Can you work these out from the model? Positions are in its coordinate system, mm. A direction names the side the tool comes from. Coordinates: 2 decimals unless noted, no trailing zeros. Write each loop counter-clockwise with the first axis right and the second up, starting at its lowest first coordinate (ties: lowest second). Pieces come first, ordered by that corner, then holes. Notation, with made-up numbers: M -21,67.5 L -1,67.5 A8 ccw -1,80.5 Z; hole C -5,1.5 d9. An arc over 180 degrees is marked long. Use one line per item in the form item = value. Start each with the question number.
```python
from build123d import *

# Parameters (mm, degrees)
SKETCH_1_W          = 70
SKETCH_1_H          = 80
EXTRUDE_1_DEPTH     = 4
SKETCH_2_W          = 70
SKETCH_2_H          = 4
EXTRUDE_2_DEPTH     = 16
CUT_EXTRUDE_1_DEPTH = 109.166538264
CHAMFER_1_SIZE      = 20
SKETCH_8_W          = 30
SKETCH_8_H          = 3
EXTRUDE_4_DEPTH     = 34
EXTRUDE_START       = 10
EXTRUDE_6_DEPTH     = 10
SKETCH_11_W         = 9
SKETCH_11_H         = 37.243398564
CUT_EXTRUDE_2_DEPTH = 10
CHAMFER_2_SIZE      = 3
SKETCH_12_W         = 3
SKETCH_12_H         = 48
EXTRUDE_7_DEPTH     = 6
CHAMFER_3_SIZE      = 5
SKETCH_13_W         = 9
SKETCH_13_H         = 3
EXTRUDE_8_DEPTH     = 6
CHAMFER_4_SIZE      = 10
CUT_EXTRUDE_3_DEPTH = 4
FILLET_3_R          = 3
SKETCH_15_R         = 2.5
CUT_EXTRUDE_4_DEPTH = 4
FILLET_4_R          = 10
SKETCH_16_R         = 1.5
CUT_EXTRUDE_5_DEPTH = 4


with BuildPart() as part:
    # 草图1 → 凸台-拉伸1 (new body)
    with BuildSketch(Plane(origin=(0, 0, 0), x_dir=(1, 0, 0), z_dir=(0, 1, 0))):
        with Locations((35, 40)):
            Rectangle(SKETCH_1_W, SKETCH_1_H)
    extrude(amount=EXTRUDE_1_DEPTH)

    # 草图2 → 凸台-拉伸2 (add)
    with BuildSketch(Plane(origin=(0, 4, 0), x_dir=(1, 0, 0), z_dir=(0, 1, 0))):
        with Locations((35, 2)):
            Rectangle(SKETCH_2_W, SKETCH_2_H)
    extrude(amount=EXTRUDE_2_DEPTH)

    # 草图4 → 切除-拉伸1 (cut, through all)
    with BuildSketch(Plane(origin=(0, 20, 0), x_dir=(1, 0, 0), z_dir=(0, 1, 0))):
        with BuildLine():
            Line((14, 29), (14, 0))
            Line((14, 0), (56, 0))
            Line((56, 0), (56, 29))
            ThreePointArc((56, 29), (35, 50), (14, 29))
        make_face()
    extrude(amount=-CUT_EXTRUDE_1_DEPTH, mode=Mode.SUBTRACT)

    # 倒角1
    chamfer_1_edges = [part.edges().sort_by_distance(p)[0] for p in [
        (0, 2, -80),
        (70, 2, -80),
    ]]
    chamfer(chamfer_1_edges, length=CHAMFER_1_SIZE)

    # 草图8 → 凸台-拉伸4 (add)
    with BuildSketch(Plane.XZ):
        with Locations((35, -78.5)):
            Rectangle(SKETCH_8_W, SKETCH_8_H)
    extrude(amount=EXTRUDE_4_DEPTH)

    # 草图10 → 凸台-拉伸6 (add)
    with BuildSketch(Plane(origin=(0, 4, 0), x_dir=(1, 0, 0), z_dir=(0, 1, 0)).offset(EXTRUDE_START)):
        with BuildLine():
            Line((42.5, 48.615045246), (42.5, 80))
            Line((42.5, 80), (27.5, 80))
            Line((27.5, 80), (27.5, 48.615045246))
            ThreePointArc((27.5, 48.615045246), (35, 50), (42.5, 48.615045246))
        make_face()
    extrude(amount=-EXTRUDE_6_DEPTH)

    # 草图11 → 切除-拉伸2 (cut)
    with BuildSketch(Plane(origin=(0, 14, 0), x_dir=(1, 0, 0), z_dir=(0, 1, 0))):
        with Locations((35, 61.378300718)):
            Rectangle(SKETCH_11_W, SKETCH_11_H)
    extrude(amount=-CUT_EXTRUDE_2_DEPTH, mode=Mode.SUBTRACT)

    # 倒角2
    chamfer_2_edges = [part.edges().sort_by_distance(p)[0] for p in [
        (35, 4, -80),
    ]]
    chamfer(chamfer_2_edges, length=CHAMFER_2_SIZE)

    # 草图12 → 凸台-拉伸7 (add)
    with BuildSketch(Plane(origin=(0, 0, -80), x_dir=(-1, 0, 0), z_dir=(0, 0, -1))):
        with Locations((-41, -10)):
            Rectangle(SKETCH_12_W, SKETCH_12_H)
        with Locations((-29, -10)):
            Rectangle(SKETCH_12_W, SKETCH_12_H)
    extrude(amount=EXTRUDE_7_DEPTH)

    # 倒角3
    chamfer_3_edges = [part.edges().sort_by_distance(p)[0] for p in [
        (41, 14, -86),
        (29, 14, -86),
    ]]
    chamfer(chamfer_3_edges, length=CHAMFER_3_SIZE)

    # 草图13 → 凸台-拉伸8 (add)
    with BuildSketch(Plane(origin=(0, 0, -80), x_dir=(-1, 0, 0), z_dir=(0, 0, -1))):
        with Locations((-35, -32.5)):
            Rectangle(SKETCH_13_W, SKETCH_13_H)
    extrude(amount=EXTRUDE_8_DEPTH)

    # 倒角4
    chamfer_4_edges = [part.edges().sort_by_distance(p)[0] for p in [
        (50, -34, -78.5),
        (20, -34, -78.5),
    ]]
    chamfer(chamfer_4_edges, length=CHAMFER_4_SIZE)

    # 草图14 → 切除-拉伸3 (cut)
    with BuildSketch(Plane(origin=(0, 4, 0), x_dir=(1, 0, 0), z_dir=(0, 1, 0))):
        Polygon((22.071067812, 75), (5, 57.928932188), (5, 36.715728753), (27.5, 59.215728753), (27.5, 75), align=None)
        Polygon((47.928932188, 75), (42.5, 75), (42.5, 59.215728753), (65, 36.715728753), (65, 57.928932188), align=None)
    extrude(amount=-CUT_EXTRUDE_3_DEPTH, mode=Mode.SUBTRACT)

    # 圆角3
    fillet_3_edges = [part.edges().sort_by_distance(p)[0] for p in [
        (47.928932188, 2, -75),
        (65, 2, -57.928932188),
        (65, 2, -36.715728753),
        (42.5, 2, -59.215728753),
        (42.5, 2, -75),
        (5, 2, -36.715728753),
        (5, 2, -57.928932188),
        (22.071067812, 2, -75),
        (27.5, 2, -75),
        (27.5, 2, -59.215728753),
    ]]
    fillet(fillet_3_edges, radius=FILLET_3_R)

    # 草图15 → 切除-拉伸4 (cut)
    with BuildSketch(Plane(origin=(0, 4, 0), x_dir=(1, 0, 0), z_dir=(0, 1, 0))):
        with Locations(Location((7, 8, 0), (0, 0, 270))):
            Circle(SKETCH_15_R)
        with Locations(Location((7, 17, 0), (0, 0, 270))):
            Circle(SKETCH_15_R)
        with Locations(Location((7, 26, 0), (0, 0, 270))):
            Circle(SKETCH_15_R)
        with Locations(Location((7, 35, 0), (0, 0, 270))):
            Circle(SKETCH_15_R)
        with Locations(Location((63, 35, 0), (0, 0, 90))):
            Circle(SKETCH_15_R)
        with Locations(Location((63, 26, 0), (0, 0, 90))):
            Circle(SKETCH_15_R)
        with Locations(Location((63, 17, 0), (0, 0, 90))):
            Circle(SKETCH_15_R)
        with Locations(Location((63, 8, 0), (0, 0, 90))):
            Circle(SKETCH_15_R)
    extrude(amount=-CUT_EXTRUDE_4_DEPTH, mode=Mode.SUBTRACT)

    # 圆角4
    fillet_4_edges = [part.edges().sort_by_distance(p)[0] for p in [
        (0, 20, -2),
        (70, 20, -2),
    ]]
    fillet(fillet_4_edges, radius=FILLET_4_R)

    # 草图16 → 切除-拉伸5 (cut)
    with BuildSketch(Plane(origin=(-162.95666402, 61.923916545, -4), x_dir=(-0.1273989198368121, 0.9918515590673908, 0), z_dir=(0, 0, -1))):
        with Locations(Location((-72.151278538, 166.87443555, 0), (0, 0, 277.319311568))):
            Circle(SKETCH_16_R)
        with Locations(Location((-78.075328311, 212.995533047, 0), (0, 0, 277.319311568))):
            Circle(SKETCH_16_R)
    extrude(amount=-CUT_EXTRUDE_5_DEPTH, mode=Mode.SUBTRACT)


solid = part.part
```
1) Which directions (+Z, -Z, +X, -X, +Y, -Y) give clear straight access to the entire face, cutting with the end or side of a thin tool? Please do faces 4 (the face through (30.5, 5, -74)), 5 (the face through (65, 2, -50)), 6 (the face through (56, 4, -43)).
2) Will these pins go through, and if not, where does the flat tip stop? pin 1 Ø3 at (x, z) = (7, -35) entering from +Y; pin 2 Ø4 at (x, y) = (46.5, -10) entering from +Z; pin 3 Ø1.8 at (x, z) = (37, -83.5) entering from +Y; pin 4 Ø3 at (x, z) = (55, -77) entering from -Y.
3) Please list where these lines run through material, in increasing order: line 1 (X direction, y = 1.9, z = -17); line 2 (Z direction, x = 63, y = 1.7); line 3 (X direction, y = 9.5, z = -58).
4) Suppose I cut it at A-A on y = 6.5. Please give me the cut outline in (x, z), and give its area (3 significant figures).
5) Suppose I cut it at D-D on z = -78. Please give me the cut outline in (x, y), and give its area (3 significant figures).
6) If we mould it in two halves opening along X, with no side actions, what happens to faces 1 (the face through (29, 11, -84)), 2 (the face through (50, -12, -79)), 3 (the face through (65.22, 2.03, -9.15))? For each: +X half, -X half, draft (parallel to the pull), parting line (faces both ways), or undercut.
7) Suppose I cut it at C-C on x = 11.75. Please give me the cut outline in (y, z).
8) Suppose I cut it at B-B on z = -8. Please give me the cut outline in (x, y).
Computed values:
q1.face_4 = -Z, +Y
q1.face_5 = +Y, -Y
q1.face_6 = -Z, +X, +Y
q2.pin_1 = through
q2.pin_2 = -77
q2.pin_3 = -31
q2.pin_4 = 0
q3.line_1 = 0 to 4.5, 9.5 to 14, 56 to 60.5, 65.5 to 70
q3.line_2 = -67 to -59.93, -41.13 to -37.5, -32.5 to -28.5, -23.5 to -19.5, -14.5 to -10.5, -5.5 to 0
q3.line_3 = 27.5 to 30.5, 39.5 to 42.5
q4.outline = M 0,-4 L 14,-4 L 14,0 L 0,0 Z; M 27.5,-86 L 30.5,-86 L 30.5,-49.51 A21 cw 27.5,-48.62 Z; M 39.5,-86 L 42.5,-86 L 42.5,-48.62 A21 cw 39.5,-49.51 Z; M 56,-4 L 70,-4 L 70,0 L 56,0 Z
q4.area = 333 mm²
q5.outline = M 18,0 L 20,0 L 20,-24 L 30,-34 L 40,-34 L 50,-24 L 50,0 L 52,0 L 52,4 L 42.5,4 L 42.5,14 L 39.5,14 L 39.5,3 L 30.5,3 L 30.5,14 L 27.5,14 L 27.5,4 L 18,4 Z
q5.area = 1,110 mm²
q6.face_1 = draft
q6.face_2 = +X half
q6.face_3 = undercut
q7.outline = M 0,-71.75 L 4,-71.75 L 4,-64.68 L 0,-64.68 Z; M 0,-43.47 L 4,-43.47 L 4,-4 L 10.12,-4 L 10.12,0 L 0,0 Z; M 13.12,-4 L 20,-4 L 20,0 L 13.12,0 Z
q8.outline = M 0,0 L 4.5,0 L 4.5,4 L 0,4 Z; M 9.5,0 L 14,0 L 14,4 L 9.5,4 Z; M 56,0 L 60.5,0 L 60.5,4 L 56,4 Z; M 65.5,0 L 70,0 L 70,4 L 65.5,4 Z
